Model file for the job. Use its own axes, mm. Face numbers are marked on the shaded views. A direction names the side the tool comes from. Round coordinates to 2 decimals unless told otherwise and drop trailing zeros. Write each loop counter-clockwise with the first axis right and the second up, starting at its lowest first coordinate (ties: lowest second). Pieces come first, ordered by that corner, then holes. Notation, with made-up numbers: (-37, 4.5) - (-25, 4.5) arc R26 ccw to (-25, 29.5) - close; hole circle Ø10 at (-27, -5). An arc over 180 degrees is marked (long way). One line per item, written item: value.
from build123d import *

# Parameters (mm, degrees)
SKETCH1_W           = 30
SKETCH1_H           = 30
SKETCH1_R           = 1
BOSS_EXTRUDE1_DEPTH = 9.144
SKETCH2_R           = 7.747
BOSS_EXTRUDE2_DEPTH = 21.844
SKETCH3_W           = 13.335
SKETCH3_H           = 3.048
BOSS_EXTRUDE3_DEPTH = 6.35


with BuildPart() as part:
    # Sketch1 → Boss-Extrude1 (new body)
    with BuildSketch(Plane(origin=(0, 0, 0), x_dir=(1, 0, 0), z_dir=(0, 1, 0))):
        with Locations((15, 15)):
            Rectangle(SKETCH1_W, SKETCH1_H)
        with Locations((28.14, 1.86)):
            Circle(SKETCH1_R, mode=Mode.SUBTRACT)
        with Locations((28.14, 28.1400088)):
            Circle(SKETCH1_R, mode=Mode.SUBTRACT)
        with Locations((1.86, 28.1400088)):
            Circle(SKETCH1_R, mode=Mode.SUBTRACT)
        with Locations((1.86, 1.86)):
            Circle(SKETCH1_R, mode=Mode.SUBTRACT)
    extrude(amount=BOSS_EXTRUDE1_DEPTH)

    # Sketch2 → Boss-Extrude2 (add)
    with BuildSketch(Plane(origin=(0, 9.144, 0), x_dir=(1, 0, 0), z_dir=(0, 1, 0))):
        with Locations((15, 15)):
            Circle(SKETCH2_R)
    extrude(amount=BOSS_EXTRUDE2_DEPTH)

    # Sketch3 → Boss-Extrude3 (add)
    with BuildSketch(Plane.XZ):
        with Locations((15, -26.19)):
            Rectangle(SKETCH3_W, SKETCH3_H)
    extrude(amount=BOSS_EXTRUDE3_DEPTH)


solid = part.part
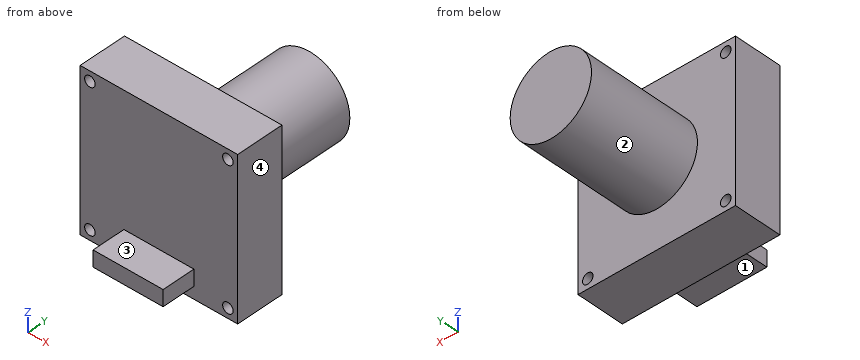
1. Wall check: probe 1 along Z at (x, y) = (1.86, 2.75); probe 2 along X at (y, z) = (2.25, -1.86); probe 3 along Z at (x, y) = (1, 9). Give the ranges that are in metal, low to high. Write a range as [from, to].
Report:
probe 1: [-30, -29.14], [-27.14, -2.86], [-0.86, 0]
probe 2: [0, 0.86], [2.86, 27.14], [29.14, 30]
probe 3: [-30, -28.65], [-27.63, -2.37], [-1.35, 0]
2. Band-saw the part on B-B on z = -1.86. Write the cut outline in (x, y), plus the area to 3 significant figures.
Report:
outline: (0, 0) - (0.86, 0) - (0.86, 9.14) - (0, 9.14) - close; (2.86, 0) - (27.14, 0) - (27.14, 9.14) - (2.86, 9.14) - close; (29.14, 0) - (30, 0) - (30, 9.14) - (29.14, 9.14) - close
area: 238 mm²
3. Band-saw the part on A-A on x = 28.14. Write the cut outline in (y, z).
Report:
outline: (0, -30) - (9.14, -30) - (9.14, -29.14) - (0, -29.14) - close; (0, -27.14) - (9.14, -27.14) - (9.14, -2.86) - (0, -2.86) - close; (0, -0.86) - (9.14, -0.86) - (9.14, 0) - (0, 0) - close
4. Drop flat-ended pins along their axis: pin 1 (0.9 mm diameter, centred on y = -4, z = -26.5, fed in from +X); pin 2 (4 mm diameter, centred on y = 16, z = -7.5, fed in from +X); pin 3 (2.5 mm diameter, centred on y = -3, z = -25.5, fed in from -X); pin 4 (12 mm diameter, centred on x = 15.5, z = -24, fed in from -Y). Give the stop position or say it passes through.
Report:
pin 1: x = 21.67
pin 2: x = 20.46
pin 3: x = 8.33
pin 4: y = -6.35
5. Band-saw the part on D-D on z = -15. Write the cut outline in (x, y).
Report:
outline: (0, 0) - (30, 0) - (30, 9.14) - (22.75, 9.14) - (22.75, 30.99) - (7.25, 30.99) - (7.25, 9.14) - (0, 9.14) - close
6. Tool access for the marked faces 1, 2, 3 and 4: list every direction of +Z, -Z, +X, -X, +Y, -Y with a clear straight run to the whole face (end or side of a thin tool).
Report:
face 1: -Z, +X, -X, -Y
face 2: +Y
face 3: +Z, +X, -X, -Y
face 4: +Z, -Z, +X, +Y, -Y
7. Band-saw the part on C-C on x = 15. Write the cut outline in (y, z).
Report:
outline: (-6.35, -27.71) - (0, -27.71) - (0, -30) - (9.14, -30) - (9.14, -22.75) - (30.99, -22.75) - (30.99, -7.25) - (9.14, -7.25) - (9.14, 0) - (0, 0) - (0, -24.67) - (-6.35, -24.67) - close
